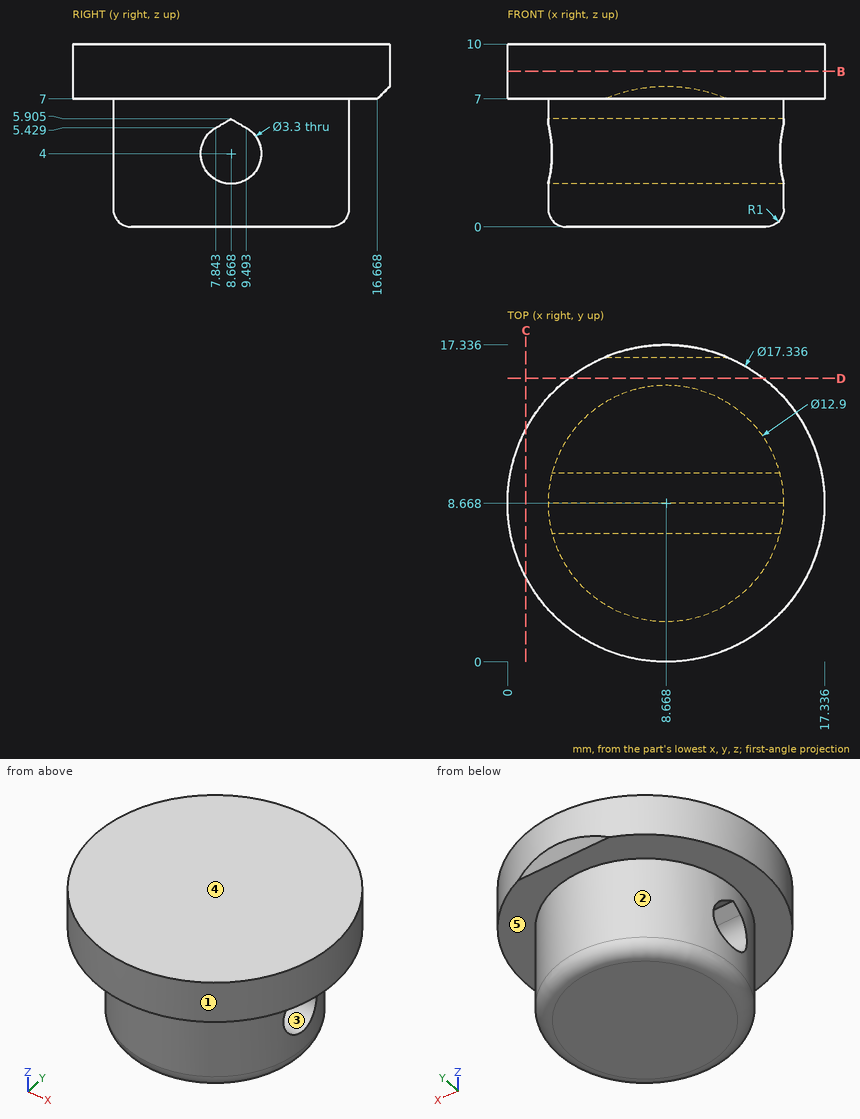
The drawing under review shows one solid part. Ordinate dimensions are in mm from its lowest x, y, z. A direction names the side the tool comes from. Coordinates: 2 decimals unless noted, no trailing zeros. Write each loop counter-clockwise with the first axis right and the second up, starting at its lowest first coordinate (ties: lowest second). Pieces come first, ordered by that corner, then holes. Notation, with made-up numbers: (51.5, 40.25) - (88.5, 40.25) arc R13 cw to (88.5, 51.25) - close; hole circle Ø10 at (71.25, 84.25). An arc over 180 degrees is marked (long way). Answer in a Markdown table with one row per item. Add a question column.
Q1. We need section C-C, the plane x = 1. State the section outline as (y, z) points.
Q2. We need section D-D, the plane y = 15.5. State the section outline as (x, z) points.
Q3. Draft analysis for pull direction Z (two halves, no side actions). For the marked faces 3, 4 and 5, state which applies: +Z half, -Z half, draft (parallel to the pull), parting line (faces both ways), or undercut.
Q4. For probe 1 along Z at (x, y) = (7.5, 2.25); probe 2 along Y at (x, z) = (9, 4); probe 3 along Z at (x, y) = (5.5, 9) (1 decimal), list the stretches that pass through material, from the lowest coordinate up.
Q5. For P1, Ø3, axis at x = 12.5, y = 3, coming from the -Z side; P2, Ø6, axis at y = 15.5, z = 8, coming from the -X side; P3, Ø5.5, axis at y = 8.67, z = 4, coming from the +X side, all flat-tipped, find the tip position at first contact; note any pin that passes through.
Q6. Tool access review of the marked faces 1 and 2: name each direction out of +Z, -Z, +X, -X, +Y, -Y from which nothing blocks a thin tool from reaching the whole face with its end or side.
Q7. We need section B-B, the plane z = 8.5. State the section outline as (x, y) points.
Answer list:
| question | item | result |
|---|---|---|
| 1 | outline | (4.63, 7) - (12.71, 7) - (12.71, 10) - (4.63, 10) - close |
| 2 | outline | (3.33, 7) - (14, 7) - (14, 10) - (3.33, 10) - close |
| 3 | face 3 | undercut |
| 3 | face 4 | +Z half |
| 3 | face 5 | -Z half |
| 4 | probe 1 | z = 7 to 10 |
| 4 | probe 2 | y = 2.23 to 7.02, 10.32 to 15.11 |
| 4 | probe 3 | z = 0 to 2.4, 5.7 to 10 |
| 5 | P1 | stops at z = 0 |
| 5 | P2 | stops at x = 0.89 |
| 5 | P3 | stops at x = 15.12 |
| 6 | face 1 | +Z, -Z |
| 6 | face 2 | -Z |
| 7 | outline | circle Ø17.34 at (8.67, 8.67) |
